```python
from build123d import *

# Parameters (mm, degrees)
SKETCH1_W                              = 60
SKETCH1_H                              = 40
BOSS_EXTRUDE1_DEPTH                    = 54
SKETCH3_W                              = 75
SKETCH3_H                              = 40
SKETCH3_R                              = 8
BOSS_EXTRUDE2_DEPTH                    = 54
CUT_EXTRUDE2_DEPTH                     = 60
TAP_DRILL_FOR_M8_HELICOIL1_D           = 8.25
TAP_DRILL_FOR_M8_HELICOIL1_CSINK_D     = 8.3
TAP_DRILL_FOR_M8_HELICOIL1_CSINK_ANGLE = 90


with BuildPart() as part:
    # Sketch1 → Boss-Extrude1 (new body)
    with BuildSketch(Plane(origin=(0, 0, 0), x_dir=(1, 0, 0), z_dir=(0, 1, 0))):
        with Locations((-30, -20)):
            Rectangle(SKETCH1_W, SKETCH1_H)
    extrude(amount=BOSS_EXTRUDE1_DEPTH)

    # Sketch3 → Boss-Extrude2 (add)
    with BuildSketch(Plane(origin=(0, 0, 0), x_dir=(1, 0, 0), z_dir=(0, 1, 0))):
        with Locations((37.5, -20)):
            Rectangle(SKETCH3_W, SKETCH3_H)
        with Locations((30, -20)):
            Circle(SKETCH3_R, mode=Mode.SUBTRACT)
    boss_extrude2 = extrude(amount=BOSS_EXTRUDE2_DEPTH)

    # Sketch4 → Cut-Extrude2 (cut)
    with BuildSketch(Plane.XY.offset(40)):
        with BuildLine():
            ThreePointArc((75, 20.458980338), (61.05699404, 11.962243847), (45, 9))
            Line((45, 9), (75, 9))
            Line((75, 9), (75, 20.458980338))
        make_face()
        with BuildLine():
            Line((45, 9), (45, 54))
            Line((45, 54), (0, 54))
            ThreePointArc((0, 54), (13.180194847, 22.180194847), (45, 9))
        make_face()
        with BuildLine():
            Line((75, 54), (45, 54))
            Line((45, 54), (45, 9))
            ThreePointArc((45, 9), (61.05699404, 11.962243847), (75, 20.458980338))
            Line((75, 20.458980338), (75, 54))
        make_face()
    cut_extrude2 = extrude(amount=-CUT_EXTRUDE2_DEPTH, mode=Mode.SUBTRACT)

    # Tap Drill for M8 Helicoil1 (through all)
    with Locations(Plane(origin=(0, 9, 0), x_dir=(1, 0, 0), z_dir=(0, 1, 0))):
        with Locations((60, -20)):
            tap_drill_for_m8_helicoil1 = CounterSinkHole(TAP_DRILL_FOR_M8_HELICOIL1_D / 2, TAP_DRILL_FOR_M8_HELICOIL1_CSINK_D / 2, counter_sink_angle=TAP_DRILL_FOR_M8_HELICOIL1_CSINK_ANGLE)

    # Mirror1: Boss-Extrude2, Cut-Extrude2, Tap Drill for M8 Helicoil1 across plane
    add(boss_extrude2.mirror(Plane(origin=(-30, 0, 0), x_dir=(0, 0, 1), z_dir=(1, 0, 0))))
    add(cut_extrude2.mirror(Plane(origin=(-30, 0, 0), x_dir=(0, 0, 1), z_dir=(1, 0, 0))), mode=Mode.SUBTRACT)
    add(tap_drill_for_m8_helicoil1.mirror(Plane(origin=(-30, 0, 0), x_dir=(0, 0, 1), z_dir=(1, 0, 0))), mode=Mode.SUBTRACT)


solid = part.part
```
Geometry: final body of the model. Coordinates: model frame, mm. A direction names the side the tool comes from. Coordinates: 2 decimals unless noted, no trailing zeros. Order: outer loops, then holes, each group sorted by start corner. A loop starts at its lowest first (then second) coordinate and runs counter-clockwise, first axis right, second up.
Item 1: Section query C-C (z = 31). Output: boundary loops of the cut face in (x, y), then the cut area to 3 significant figures.
Answer:
outline: (-135, 0) - (75, 0) - (75, 9) - (45, 9) arc R45 cw to (0, 54) - (-60, 54) arc R45 cw to (-105, 9) - (-135, 9) - close
area: 5,460 mm2
Item 2: Section query B-B (z = 20). Output: boundary loops of the cut face in (x, y) (3 decimals), then the cut area to 3 significant figures.
Answer:
outline: (-135, 0) - (-124.125, 0) - (-124.125, 8.975) - (-124.15, 9) - (-135, 9) - close; (-115.875, 0) - (-98, 0) - (-98, 9.548) arc R45 cw to (-105, 9) - (-115.85, 9) - (-115.875, 8.975) - close; (-82, 0) - (22, 0) - (22, 15.322) arc R45 cw to (0, 54) - (-60, 54) arc R45 cw to (-82, 15.322) - close; (38, 0) - (55.875, 0) - (55.875, 8.975) - (55.85, 9) - (45, 9) arc R45 cw to (38, 9.548) - close; (64.125, 0) - (75, 0) - (75, 9) - (64.15, 9) - (64.125, 8.975) - close
area: 4,930 mm2
Item 3: Contact query for flat-ended pins moving along their axis: P1, Ø13, axis at x = -90, z = 20, coming from the +Y side; P2, Ø3, axis at y = 26.5, z = 28.5, coming from the +X side; P3, Ø5, axis at y = 26, z = 5.5, coming from the +X side; P4, Ø8, axis at y = 38, z = 12, coming from the -X side. Output: stop coordinate, or through.
Answer:
P1: passes through
P2: stops at x = 10.59
P3: stops at x = 11.91
P4: stops at x = -64.69
Item 4: Section query D-D (x = 30). Output: boundary loops of the cut face in (y, z), then the cut area to 3 significant figures.
Answer:
outline: (0, 0) - (11.57, 0) - (11.57, 12) - (0, 12) - close; (0, 28) - (11.57, 28) - (11.57, 40) - (0, 40) - close
area: 278 mm2
Item 5: Access query for faces 4 (the face through (-120, 9, 25)), 5 (the face through (-29, 0, 20)). Directions: +Z, -Z, +X, -X, +Y, -Y. A direction counts if a zero-diameter tool reaches every point of the face in a straight line with its end or side. Return the directions, or none.
Answer:
face 4: +Z, -Z, -X, +Y
face 5: +Z, -Z, +X, -X, -Y
Item 6: Draft query along Z for faces 1 (the face through (60, 9, 25)), 2 (the face through (-82, 6, 20)), 3 (the face through (-29, 21, 40)). Return one class per face: released by +Z, released by -Z, zero draft, split by the parting line, or undercut.
Answer:
face 1: zero draft
face 2: undercut
face 3: released by +Z
Item 7: Material intervals for line 1 along Z through (x, y) = (-90, 11.25); line 2 along Y through (x, z) = (58, 11.5); line 3 along Z through (x, y) = (60, 5.5) (3 decimals), sorted ascending.
Answer:
line 1: z = 0 to 12, 28 to 40
line 2: y = 0 to 9
line 3: z = 0 to 15.875, 24.125 to 40
Item 8: Section query A-A (x = 60). Output: boundary loops of the cut face in (y, z) (3 decimals), then the cut area to 3 significant figures.
Answer:
outline: (0, 0) - (9, 0) - (9, 15.85) - (8.975, 15.875) - (0, 15.875) - close; (0, 24.125) - (8.975, 24.125) - (9, 24.15) - (9, 40) - (0, 40) - close
area: 286 mm2
